The listing builds one solid part. Answer for the finished solid, in the listing's coordinates (mm). A direction names the side the tool comes from. Give positions to 0.01 mm unless a question says otherwise; leave off trailing zeros. Order: outer loops, then holes, each group sorted by start corner. A loop starts at its lowest first (then second) coordinate and runs counter-clockwise, first axis right, second up. Notation, with made-up numbers: (81.5, 76.25) -> (120.5, 76.25) arc R19 cw to (120.5, 93.25) -> close; hole circle Ø2 at (17, 82.25). An arc over 180 degrees is marked (long way). One line per question, with ' | ' between items. Start each with the question number.
```python
from build123d import *

# Parameters (mm, degrees)
EXTRUDE_1_DEPTH = 3.2
SKETCH_2_R      = 2
EXTRUDE_2_DEPTH = 80
FILLET_1_R      = 0.16


with BuildPart() as part:
    # 草图1 → 凸台-拉伸1 (new body)
    with BuildSketch(Plane.XY):
        Polygon((0, 4.041451884), (-3.5, 2.020725942), (-3.5, -2.020725942), (0, -4.041451884), (3.5, -2.020725942), (3.5, 2.020725942), align=None)
    extrude(amount=-EXTRUDE_1_DEPTH)

    # 草图3 → 切除-旋转1 (revolve, cut)
    with BuildSketch(Plane(origin=(0, 0, 0), x_dir=(0, 0, -1), z_dir=(1, 0, 0))):
        Polygon((0.523, 4.041451884), (0, 3.518451884), (0, 4.041451884), align=None)
        Polygon((3.2, 4.041451884), (3.2, 3.518451884), (2.677, 4.041451884), align=None)
    revolve(axis=Axis((0, 0, 0), (0, 0, 1)), mode=Mode.SUBTRACT)

    # 草图2 → 凸台-拉伸2 (add)
    with BuildSketch(Plane.XY):
        Circle(SKETCH_2_R)
    extrude(amount=EXTRUDE_2_DEPTH)

    # 圆角1
    fillet_1_edges = [part.edges().sort_by_distance(p)[0] for p in [
        (-2, 0, 80),
    ]]
    fillet(fillet_1_edges, radius=FILLET_1_R)


solid = part.part
```
(1) For faces 1 (the face through (2, -2, 0)), 2 (the face through (-1.8, -3, -1.6)), determine the directions among +Z, -Z, +X, -X, +Y, -Y from which every point of the face is accessible in a straight line to the end or side of a thin tool.
(2) Given P1, Ø1, axis at x = -2, z = 22.5, coming from the -Y side; P2, Ø3, axis at x = 1.5, y = 3, coming from the +Z side; P3, Ø2, axis at x = 2.5, z = 52, coming from the +Y side; P4, Ø1.5, axis at y = 1, z = 62, coming from the -X side, each flat-ended and moving along its own axis, determine where each tip first touches the part or whether it passes through.
(3) The part is cut by section A-A on z = 61. Determine the outline of the cut face in (x, y).
(4) Consider line 1 (Z direction, x = -2.25, y = -1.25); line 2 (Y direction, x = -0.75, z = 39); line 3 (X direction, y = 0.5, z = 35). Determine where each line is inside the solid, lowest interval first.
Result sheet:
1) face 1: +Z | face 2: +Z, -Z, -X, -Y
2) P1: stops at y = -1.32 | P2: stops at z = 80 | P3: stops at y = 1.32 | P4: stops at x = -1.98
3) outline: circle Ø4 at (0, 0)
4) line 1: z = -3.2 to 0 | line 2: y = -1.85 to 1.85 | line 3: x = -1.94 to 1.94
